Input: part model. Units: mm. Frame: model coordinates. Coordinates: 2 decimals unless noted, no trailing zeros. Order: outer loops, then holes, each group sorted by start corner. A loop starts at its lowest first (then second) coordinate and runs counter-clockwise, first axis right, second up. Notation, with made-up numbers: (29.25, 36) - (54.25, 36) arc R18 cw to (54.25, 55) - close; hole circle Ø11 at (59.25, -11.5). An arc over 180 degrees is marked (long way). One line per question, with ' | ' between items.
Autodesk Fusion 360 part; units mm, degrees
sketch "Sketch1" plane through (0, 0, 0) normal (1, 0, 0) x (0, 1, 0)
  line L0 (-8, 0) -> (8, 0)
  line L1 (8, 0) -> (8, 12)
  line L2 (8, 12) -> (6, 12)
  line L3 (-8, 0) -> (-8, 12)
  line L4 (-8, 12) -> (-6, 12)
  line L5 (6, 12) -> (6, 2)
  line L6 (6, 2) -> (-6, 2)
  line L7 (-6, 2) -> (-6, 12)
  dimension "d26" = 16
  dimension "d27" = 12
  dimension "d28" = 2
  dimension "d29" = 12
  dimension "d30" = 2
  dimension "d31" = 10
  dimension "d32" = 12
  dimension "d33" = 10
sketch "Sketch2" plane through (0, 0, 1.3) normal (0, 0, 1) x (-1, 0, 0)
  line L0 (800, 3) -> (-800, 3)
  line L1 (-800, 3) -> (-800, -3)
  line L2 (-800, -3) -> (800, -3)
  line L3 (800, -3) -> (800, 3)
  line L4 (800, 0) -> (792, 0) construction
  circle A0 centre (792, 0) radius 2
  line L5 (792, 0) -> (750, 0) construction
  circle A1 centre (750, 0) radius 2
  line L6 (-800, 0) -> (-792, 0) construction
  circle A2 centre (-792, 0) radius 2
  line L7 (-792, 0) -> (-750, 0) construction
  circle A3 centre (-750, 0) radius 2
  dimension "d14" = 8
  dimension "d15" = 4
  dimension "d16" = 42
  dimension "d17" = 4
  dimension "d18" = 8
  dimension "d19" = 4
  dimension "d20" = 42
  dimension "d21" = 4
extrude "Extrude3" add sketch "Sketch1" along normal mid plane 1600
extrude "Extrude4" cut sketch "Sketch2" along normal blind 0.7 and the other way blind 1.3 contours A0 | A1 | A2 | A3
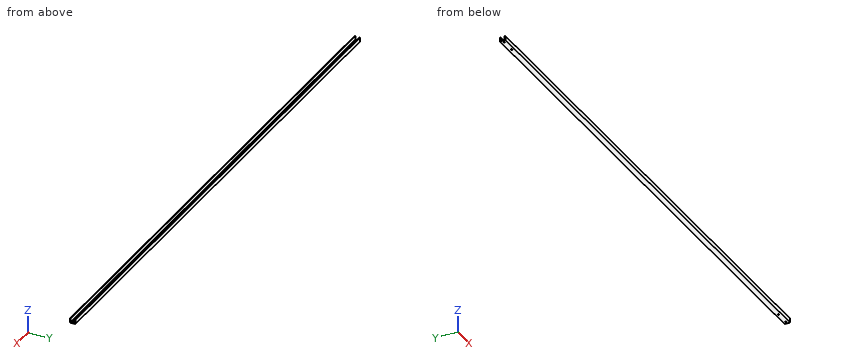
Item 1: Contact query for a flat-ended pin moving along its axis: P1, Ø1.5, axis at x = -310.5, y = 4, coming from the +Z side. Output: stop coordinate, or through.
Data:
P1: z = 2
Item 2: Section A-A on z = 8.75. Return the cut outline in (x, y), and give its area (3 significant figures).
Data:
outline: (-800, -8) - (800, -8) - (800, -6) - (-800, -6) - close; (-800, 6) - (800, 6) - (800, 8) - (-800, 8) - close | area: 6,400 mm^2
Item 3: Section B-B on x = -351. Return the cut outline in (y, z), and give its area (3 significant figures).
Data:
outline: (-8, 0) - (8, 0) - (8, 12) - (6, 12) - (6, 2) - (-6, 2) - (-6, 12) - (-8, 12) - close | area: 72.0 mm^2
Item 4: Ray query, line 1 (X direction, y = 0, z = 0.5); line 2 (X direction, y = 0.5, z = 1); line 3 (Y direction, x = 680, z = 8.25). Return the intervals inside material, ascending.
Data:
line 1: -800 to -794, -790 to -752, -748 to 748, 752 to 790, 794 to 800 | line 2: -800 to -793.94, -790.06 to -751.94, -748.06 to 748.06, 751.94 to 790.06, 793.94 to 800 | line 3: -8 to -6, 6 to 8
